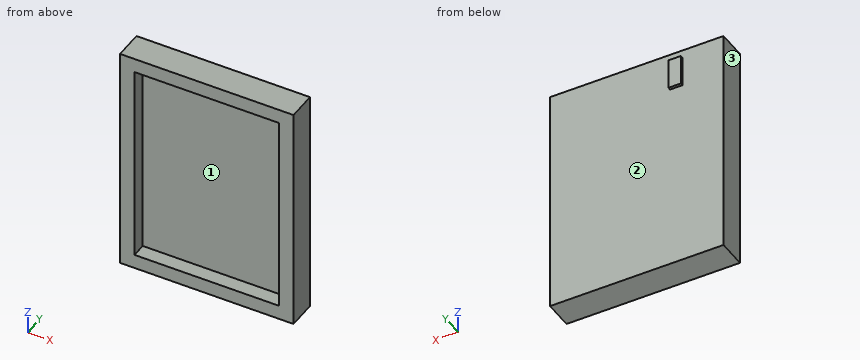
Autodesk Inventor part; units mm, degrees
ref_plane "Work Plane1" through (-600, 0, -150) normal (0, 0, 1) x (1, 0, 0)
ref_plane "Work Plane2" through (-150, 0, 0) normal (1, 0, 0) x (0, 0, -1)
ref_plane "YZ Plane" through (0, 0, 0) normal (1, 0, 0) x (0, 1, 0)
sketch "Sketch1" plane through (0, 0, 0) normal (0, 1, 0) x (-1, 0, 0)
  line L0 (0, 0) -> (600, 0)
  line L1 (600, 0) -> (600, -800)
  line L2 (600, -800) -> (0, -800)
  line L3 (0, -800) -> (0, 0)
  line L4 (0, 0) -> (0, -50)
  line L5 (0, -50) -> (50, -50)
  line L6 (50, -50) -> (550, -50)
  line L7 (550, -50) -> (550, -750)
  line L8 (550, -750) -> (50, -750)
  line L9 (50, -750) -> (50, -50)
  dimension "d0" = 600
  dimension "d1" = 800
  dimension "d2" = 50
  dimension "d3" = 50
  dimension "d4" = 50
  dimension "d5" = 50
extrude "Extrusion1" add sketch "Sketch1" along normal blind 100 contours L6 L7 L8 L9 | L0 L1 L2 L3
extrude "Extrusion2" cut sketch "Sketch1" along normal blind 50 contours L6 L7 L8 L9
sketch "Sketch2" plane through (0, 100, 0) normal (0, 1, 0) x (1, 0, 0)
  line L0 (-600, 800) -> (-600, 0)
  line L1 (-600, 800) -> (-600, 700)
  line L2 (-600, 700) -> (-400, 700)
  arc A0 (-337.5, 762.5) -> (-337.5, 637.5) centre (-337.5, 700) ccw
  line L3 (-337.5, 762.5) -> (-50, 762.5)
  line L4 (-50, 750) -> (-550, 750)
  line L5 (-50, 762.5) -> (-50, 162.5)
  line L6 (-50, 50) -> (-50, 750)
  line L7 (-337.5, 637.5) -> (-175, 637.5)
  line L8 (-175, 637.5) -> (-175, 162.5)
  line L9 (0, 800) -> (-600, 800)
  point P0 (0, 0)
  dimension "d10" = 100
  dimension "d11" = 200
  dimension "d12" = 125
  dimension "d13" = 62.5
  dimension "d14" = 600
  dimension "d15" = 125
  dimension "d16" = 100
  dimension "d17" = 287.5
  dimension "d18" = 475
  dimension "d19" = 125
ref_plane "Work Plane1" through (-600, 0, -150) normal (0, 0, 1) x (1, 0, 0)
sketch "Sketch5" plane through (0, 0, 0) normal (1, 0, 0) x (0, 0, -1)
  point P0 (0, 0)
ref_plane "Work Plane2" through (-150, 0, 0) normal (1, 0, 0) x (0, 0, -1)
sketch "Sketch10" plane through (0, 100, 0) normal (0, 1, 0) x (1, 0, 0)
  line L0 (-458, 28) -> (-415, 28)
  line L1 (-415, 28) -> (-415, 133)
  line L2 (-415, 133) -> (-458, 133)
  line L3 (-458, 133) -> (-458, 28)
  point P0 (0, 0)
extrude "Extrusion9" add sketch "Sketch10" along normal blind 10
sketch "Sketch11" plane through (-415, 100, -133) normal (0, 0, -1) x (-1, 0, 0)
  circle A0 centre (21, 4) radius 0.5
  point P0 (-415, -100)
  dimension "d46" = 1
extrude "Extrusion10" cut sketch "Sketch11" against normal through all
properties part number "base"
Geometry check sheet. Reference: the model listing, model coordinates, mm. Face numbers are marked on the shaded views. Give positions to 0.01 mm unless a question says otherwise; leave off trailing zeros. Order: outer loops, then holes, each group sorted by start corner. A loop starts at its lowest first (then second) coordinate and runs counter-clockwise, first axis right, second up.
1) Cross-section at C-C (x = -125). Record the boundary of the cut face in (y, z), then the cut area to 3 significant figures.
Results are:
outline: (0, -800) - (100, -800) - (100, 0) - (0, 0) - (0, -50) - (50, -50) - (50, -750) - (0, -750) - close
area: 45,000 mm2
2) Material ranges on probe 1 along Y at (x, z) = (-436, -68); probe 2 along X at (y, z) = (28, -407); probe 3 along Y at (x, z) = (-558, -576.5), recorded low to high.
Results are:
probe 1: y = 50 to 103.5, 104.5 to 110
probe 2: x = -600 to -550, -50 to 0
probe 3: y = 0 to 100
3) Gauge pin test, flat ends, axial feed: pin 1 (2 mm diameter, centred on x = -96, z = -323, fed in from +Y); pin 2 (12 mm diameter, centred on x = -357.5, z = -681, fed in from -Y); pin 3 (3 mm diameter, centred on x = -427, y = 107, fed in from +Z). Record the tip position at first contact, or that the pin passes through.
Results are:
pin 1: stops at y = 100
pin 2: stops at y = 50
pin 3: stops at z = -28
4) Cross-section at B-B (z = -113). Record the boundary of the cut face in (x, y), then the cut area to 3 significant figures.
Results are:
outline: (-600, 0) - (-550, 0) - (-550, 50) - (-50, 50) - (-50, 0) - (0, 0) - (0, 100) - (-415, 100) - (-415, 110) - (-458, 110) - (-458, 100) - (-600, 100) - close; hole circle Ø1 at (-436, 104)
area: 35,400 mm2
5) Cross-section at A-A (y = 9.5). Record the boundary of the cut face in (x, z), then the cut area to 3 significant figures.
Results are:
outline: (-600, -800) - (0, -800) - (0, 0) - (-600, 0) - close; hole (-550, -750) - (-50, -750) - (-50, -50) - (-550, -50) - close
area: 130,000 mm2
6) Draft check along X on the marked faces 1, 2 and 3. Enter one of: released by +X, released by -X, zero draft, split by the parting line, or undercut.
Results are:
face 1: undercut
face 2: zero draft
face 3: released by -X
